Source: CAD feature listing. Evaluate the final solid. Frame: model axes, mm. Face numbers are marked on the shaded views. A direction names the side the tool comes from. Give positions to 0.01 mm unless a question says otherwise; leave off trailing zeros. Loops run counter-clockwise (first coordinate to the right, second up) from the corner with the lowest first, then second, coordinate; pieces in that order, holes last. Notation, with made-up numbers: (69, -7.75) -> (123, -7.75) arc R19 cw to (123, 14.25) -> close; hole circle Ø5 at (-25.75, -38). An arc over 180 degrees is marked (long way). Put each result on its own line as item: value.
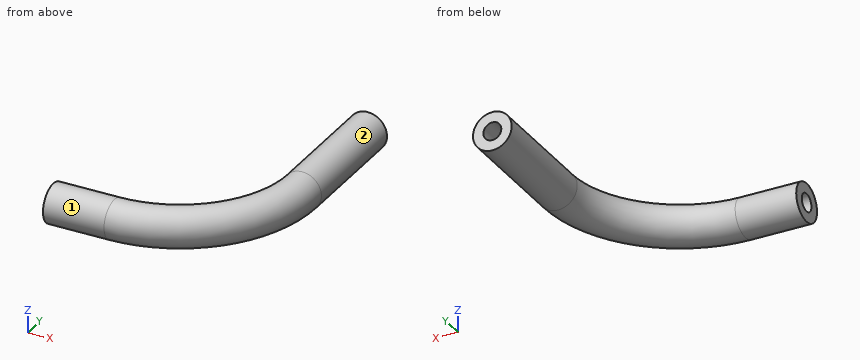
```python
from build123d import *

# Parameters (mm, degrees)
SWEEP_SOTTILE1_PROFILE_R   = 1.585
SWEEP_SOTTILE1_PROFILE_R_2 = 0.735


with BuildPart() as part:
    # Sweep-Sottile1: sweep along a curve in space
    with BuildLine() as sweep_sottile1_path:
        Line((0, 20, 0), (0, 10, 0))
        ThreePointArc((0, 10, 0), (-2.928932188, 2.928932188, 0), (-10, 0, 0))
        Line((-10, 0, 0), (-15, 0, 0))
    # Sweep-Sottile1 profile (on start of the path) → Sweep-Sottile1 (sweep)
    with BuildSketch(Plane(origin=(0, 20, 0), x_dir=(0, 0, -1), z_dir=(0, -1, 0))):
        Circle(SWEEP_SOTTILE1_PROFILE_R)
        Circle(SWEEP_SOTTILE1_PROFILE_R_2, mode=Mode.SUBTRACT)
    sweep(path=sweep_sottile1_path.line)


solid = part.part
```
(1) Line query: probe 1 along X at (y, z) = (12.5, 0) (3 decimals). Output: solid intervals per line, ascending. Write a range as from..to.
Calculated:
probe 1: x = -1.585..-0.735, 0.735..1.585
(2) First-contact query: P1, Ø1.2, axis at y = 0, z = 0, coming from the +X side; P2, Ø1, axis at y = 5.5, z = 1, coming from the +X side; P3, Ø1.2, axis at x = 0, z = 0, coming from the -Y side. Flat tips, straight axial feed; report the tip coordinate or a pass-through.
Calculated:
P1: stops at x = -3.23
P2: stops at x = 0.67
P3: stops at y = 3.23
(3) Section A-A on z = 0. Return loops of the section in (x, y) (3 decimals).
Calculated:
outline: (-15, -1.585) -> (-10, -1.585) arc R11.585 ccw to (1.585, 10) -> (1.585, 20) -> (0.735, 20) -> (0.735, 10) arc R10.735 cw to (-10, -0.735) -> (-15, -0.735) -> close; (-15, 0.735) -> (-10, 0.735) arc R9.265 ccw to (-0.735, 10) -> (-0.735, 20) -> (-1.585, 20) -> (-1.585, 10) arc R8.415 cw to (-10, 1.585) -> (-15, 1.585) -> close
(4) Reachability of the marked faces 1 and 2 from +Z, -Z, +X, -X, +Y, -Y: full face, straight path, thin tool, end or side. Return the list, or none.
Calculated:
face 1: -X
face 2: +Y
(5) Section D-D on z = 1.2. Return loops of the section in (x, y), then the cut area to 3 significant figures.
Calculated:
outline: (-15, -1.04) -> (-10, -1.04) arc R11.04 ccw to (1.04, 10) -> (1.04, 20) -> (-1.04, 20) -> (-1.04, 10) arc R8.96 cw to (-10, 1.04) -> (-15, 1.04) -> close
area: 63.6 mm²
(6) Section B-B on x = -12.5. Return loops of the section in (y, z) (3 decimals).
Calculated:
outline: circle Ø3.17 at (0, 0); hole circle Ø1.47 at (0, 0)
